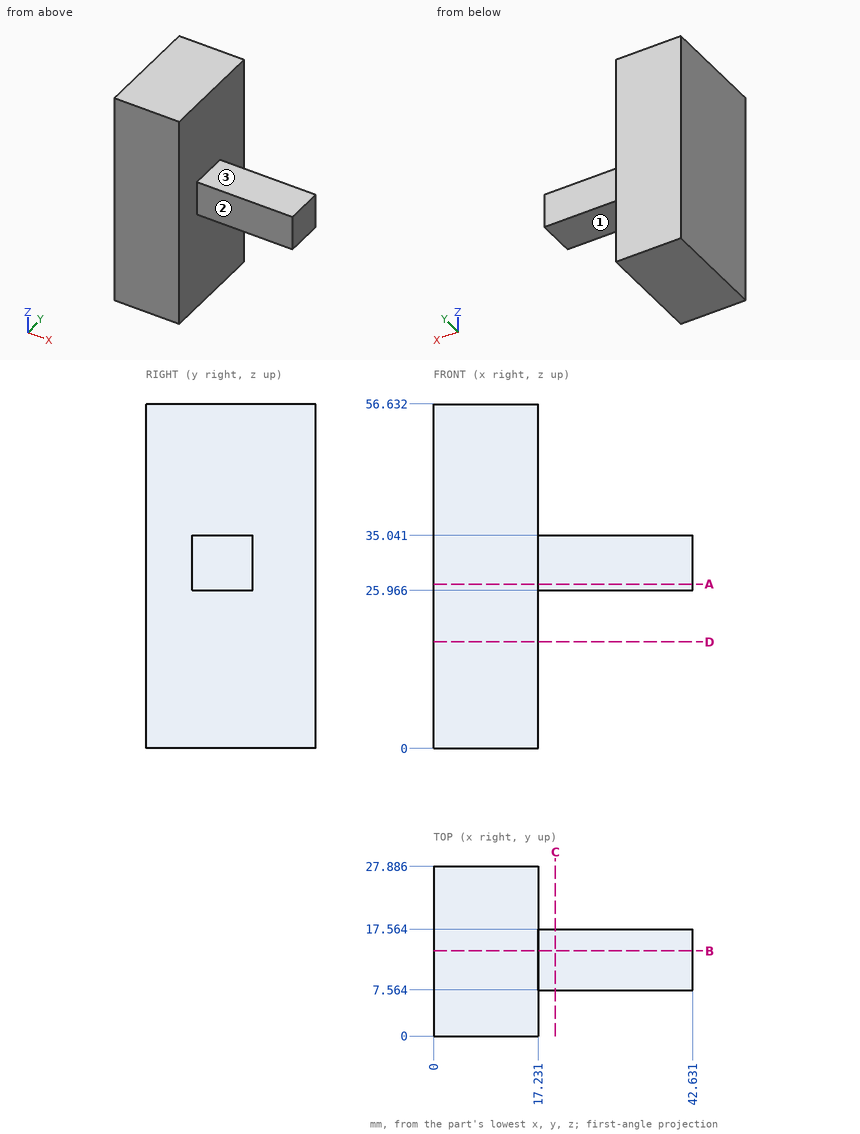
Job drawing, mm, ordinate dimensions from the low corner. One solid piece. A direction names the side the tool comes from. Round coordinates to 2 decimals unless told otherwise and drop trailing zeros. Loops run counter-clockwise (first coordinate to the right, second up) from the corner with the lowest first, then second, coordinate; pieces in that order, holes last. Notation, with made-up numbers: (2.5, -33.5) -> (51.5, -33.5) arc R31 ccw to (51.5, -1.5) -> close; hole circle Ø4 at (7, -17.75). An arc over 180 degrees is marked (long way). Use CSV: the item, a comma, the result in double quotes. Start each with the question number.
Q1. Saw through at C-C on x = 20. Give the cut face in (y, z).
Q2. Drill centre lines: L1, parallel to X at y = 4, z = 7; L2, parallel to Z at x = 40.5, y = 17.5; L3, parallel to Y at x = 24, z = 30.5. Where is each one in solid material? Low to high.
Q3. Saw through at B-B on y = 14. Give the cut face in (x, z).
Q4. Saw through at A-A on z = 27. Give the cut face in (x, y).
Q5. Saw through at D-D on z = 17.5. Give the cut face in (x, y).
Q6. Which spindle directions (+Z, -Z, +X, -X, +Y, -Y) get a long thin tool onto all of the face, cutting with end or side? Do the marked faces 1, 2 and 3. Say none if no direction does.
Q7. Flat gauge pins, fed straight in: pin 1 Ø7.5 at (x, z) = (31.5, 30.5) entering from -Y; pin 2 Ø3 at (y, z) = (17.5, 47.5) entering from +X; pin 3 Ø3 at (x, y) = (31.5, 15) entering from +Z; pin 4 Ø1 at (x, y) = (34, 6.5) entering from +Z. Where does each tip first touch, or does it go through?
Solutions:
1,outline,"(7.56, 25.97) -> (17.56, 25.97) -> (17.56, 35.04) -> (7.56, 35.04) -> close"
2,L1,"x = 0 to 17.23"
2,L2,"z = 25.97 to 35.04"
2,L3,"y = 7.56 to 17.56"
3,outline,"(0, 0) -> (17.23, 0) -> (17.23, 25.97) -> (42.63, 25.97) -> (42.63, 35.04) -> (17.23, 35.04) -> (17.23, 56.63) -> (0, 56.63) -> close"
4,outline,"(0, 0) -> (17.23, 0) -> (17.23, 7.56) -> (42.63, 7.56) -> (42.63, 17.56) -> (17.23, 17.56) -> (17.23, 27.89) -> (0, 27.89) -> close"
5,outline,"(0, 0) -> (17.23, 0) -> (17.23, 27.89) -> (0, 27.89) -> close"
6,face 1,"-Z, +X, +Y, -Y"
6,face 2,"+Z, -Z, +X, -Y"
6,face 3,"+Z, +X, +Y, -Y"
7,pin 1,"stops at y = 7.56"
7,pin 2,"stops at x = 17.23"
7,pin 3,"stops at z = 35.04"
7,pin 4,"passes through"
